Here's how the part is built. I have some questions about the finished solid (model axes, mm). Round coordinates to 2 decimals unless told otherwise and drop trailing zeros. Loops run counter-clockwise (first coordinate to the right, second up) from the corner with the lowest first, then second, coordinate; pieces in that order, holes last. Notation, with made-up numbers: M -2,38.5 L 39,38.5 A29 cw 39,69.5 Z; hole C 72,68 d1. An arc over 180 degrees is marked long. Answer as a JSON object with one key per item and string values.
Autodesk Inventor part; units mm, degrees
ref_plane "Work Plane2" through (-25, 40, 8) normal (0, -1, 0) x (1, 0, 0)
ref_plane "YZ Plane" through (0, 0, 0) normal (1, 0, 0) x (0, 1, 0)
ref_plane "XZ Plane" through (0, 0, 0) normal (0, 1, 0) x (-1, 0, 0)
sketch "Sketch1" plane through (0, 0, 0) normal (0, 0, 1) x (1, 0, 0)
  line L0 (-25, 0) -> (25, 0)
  line L1 (25, 0) -> (25, 80)
  line L2 (25, 80) -> (-25, 80)
  line L3 (-25, 80) -> (-25, 0)
  point P0 (0, 0)
  point P1 (0, 0)
  dimension "d2" = 80
  dimension "d3" = 50
extrude "Plate1" add sketch "Sketch1" along normal blind 8
hole "Hole1" at (0, 65, 8) direction (0, 0, -1) diameter 8.376 depth 8 tip angle 118
ref_plane "Work Plane1" through (0, 0, 8) normal (-1, 0, 0) x (0, 0, 1)
ref_plane "Work Plane2" through (-25, 40, 8) normal (0, -1, 0) x (1, 0, 0)
mirror "Mirror1" about plane through (-25, 40, 8) normal (0, -1, 0) of "Hole1"
fillet "Corner Round1" radius 1 4 edges at (-25, 0, 4) (25, 0, 4) (-25, 80, 4) (25, 80, 4)
equation "\"d12\" = Thickness"
equation "\"BendReliefWidth\" = Thickness"
equation "\"CornerReliefSize\" = 4 * Thickness"
equation "\"MinimumRemnant\" = 2 * Thickness"
equation "\"TransitionRadius\" = BendRadius"
equation "\"d4\" = BendRadius"
equation "\"JacobiRadiusSize\" = Thickness"
equation "\"GapSize\" = Thickness"
properties part number "draadlat poot" material "Steel, Mild"
Item 1: I want a section at C-C on z = 6.25. List the corners of the cut face in (x, y) for me.
Solution:
{"outline": "M -25,1 A1 ccw -24,0 L 24,0 A1 ccw 25,1 L 25,79 A1 ccw 24,80 L -24,80 A1 ccw -25,79 Z; hole C 0,15 d8.38; hole C 0,65 d8.38"}
Item 2: For P1, Ø8, axis at x = -20, y = 14, coming from the -Z side, with a flat end and sliding along its axis, tell me the tip position at first contact or that it passes through.
Solution:
{"P1": "stops at z = 0"}
Item 3: If I drill on L1, parallel to Y at x = 0, z = 6.75; L2, parallel to X at y = 15, z = 2.25; L3, parallel to X at y = 66, z = 7, over which ranges is the centre line in solid material (lowest first)? Write a range as from..to.
Solution:
{"L1": "y = 0..10.81, 19.19..60.81, 69.19..80", "L2": "x = -25..-4.19, 4.19..25", "L3": "x = -25..-4.07, 4.07..25"}
Item 4: I want a section at A-A on y = 15. List the corners of the cut face in (x, z) for me, plus the area to 3 significant figures.
Solution:
{"outline": "M -25,0 L -4.19,0 L -4.19,8 L -25,8 Z; M 4.19,0 L 25,0 L 25,8 L 4.19,8 Z", "area": "333 mm2"}
Item 5: We'd pull the mould along Y, two halves only. Please class faces 1 (the face through (0, 0, 4)), 2 (the face through (-25, 41, 4)), 3 (the face through (-1.258, 61.005, 3.944)), 4 (the face through (1.258, 18.995, 3.944)): +Y half, -Y half, draft (parallel to the pull), parting line (faces both ways), or undercut.
Solution:
{"face 1": "-Y half", "face 2": "draft", "face 3": "undercut", "face 4": "undercut"}
Item 6: I want a section at B-B on x = 0. List the corners of the cut face in (y, z) for me, plus the area to 3 significant figures.
Solution:
{"outline": "M 0,0 L 10.81,0 L 10.81,8 L 0,8 Z; M 19.19,0 L 60.81,0 L 60.81,8 L 19.19,8 Z; M 69.19,0 L 80,0 L 80,8 L 69.19,8 Z", "area": "506 mm2"}
